Design review of the part built by this model. Coordinates are the model's own, in mm. A direction names the side the tool comes from. Round coordinates to 2 decimals unless told otherwise and drop trailing zeros. Order: outer loops, then holes, each group sorted by start corner. A loop starts at its lowest first (then second) coordinate and runs counter-clockwise, first axis right, second up.
from build123d import *

# Parameters (mm, degrees)
BOSS_EXTRUDE1_DEPTH = 177.8
CUT_EXTRUDE1_REACH  = 236.418
SKETCH3_W           = 0.7874
SKETCH3_H           = 5.8674
FILLET1_R           = 0.15875


with BuildPart() as part:
    # Sketch1 → Boss-Extrude1 (new body)
    with BuildSketch(Plane.XY):
        with BuildLine():
            Line((151.898604, 0.02286), (152.4, 0))
            add(Edge.make_bspline(
                [(152.4, 0), (152.232833718, 0.018502415), (151.571843934, 0.091662545), (150.113999557, 0.2838596), (147.749385864, 0.638650629), (144.555943786, 1.170157002), (140.615360499, 1.859099247), (136.007834995, 2.67146013), (130.806388019, 3.562840017), (125.073826155, 4.486154777), (118.864690135, 5.397753278), (112.233312125, 6.272974236), (105.243489487, 7.106058892), (97.969665406, 7.889319693), (90.492724993, 8.606734858), (82.895253241, 9.240670251), (75.258667902, 9.77749908), (67.662928423, 10.198815718), (60.186827499, 10.49170102), (52.905945954, 10.645080099), (45.891743713, 10.644551806), (39.210681048, 10.486247597), (32.923263797, 10.164412711), (27.083700854, 9.670939726), (21.73719754, 9.016508091), (16.924344759, 8.204081974), (12.676275305, 7.249770479), (9.019815693, 6.174457771), (5.965694819, 5.002018522), (3.544032537, 3.769871526), (1.704834708, 2.531499726), (0.575239506, 1.344737529), (-0.170728015, 0.20310696), (0.337603285, -1.001772228), (1.792943226, -1.546726795), (3.794232235, -2.17716446), (6.643400201, -2.643922316), (10.216110654, -3.041953632), (14.530084187, -3.319872228), (19.533969629, -3.497677255), (25.18692206, -3.577638345), (31.428627275, -3.573848082), (38.191948203, -3.496581442), (45.401595317, -3.349308986), (52.97841726, -3.141841288), (60.83867414, -2.885262261), (68.894988424, -2.587930905), (77.057432025, -2.258882887), (85.235009672, -1.907730283), (93.335426834, -1.550168819), (101.266049649, -1.195465221), (108.93417081, -0.862411006), (116.2464986, -0.557504045), (123.110150899, -0.306936183), (129.431690533, -0.107922528), (135.123521438, 0.027974451), (140.103603919, 0.108900525), (144.29941542, 0.13993859), (147.644768246, 0.124243061), (150.083437285, 0.086502888), (151.399782071, 0.04034956), (151.898604, 0.02286)],
                knots=[0, 0, 0, 0, 0.001635356, 0.006466337, 0.014296592, 0.024884209, 0.037943993, 0.053194137, 0.070376569, 0.089257218, 0.109651763, 0.131396199, 0.15429467, 0.178096903, 0.202530723, 0.227328973, 0.252225807, 0.276966075, 0.301296827, 0.324972089, 0.347773046, 0.369493849, 0.389946985, 0.408979416, 0.42646579, 0.442306729, 0.45642124, 0.468773538, 0.47934515, 0.488155641, 0.495223141, 0.500608248, 0.504417036, 0.507344225, 0.511892731, 0.518766333, 0.5280624, 0.539750485, 0.553781924, 0.570059197, 0.588441486, 0.608747967, 0.630750044, 0.65420771, 0.678865071, 0.70445057, 0.730677503, 0.757253937, 0.783882587, 0.810265561, 0.836095192, 0.861073222, 0.884896986, 0.907258357, 0.92785625, 0.946394646, 0.962618154, 0.976286171, 0.987192828, 0.99514679, 1, 1, 1, 1], degree=3))
        make_face()
    extrude(amount=BOSS_EXTRUDE1_DEPTH)

    # Sketch3 → Cut-Extrude1 (cut, up to next)
    with BuildSketch(Plane.XY.offset(177.8), mode=Mode.PRIVATE) as cut_extrude1_sk1:
        with BuildLine():
            Line((76.2, -2.290863726), (76.2, 9.698555773))
            add(Edge.make_bspline(
                [(76.2, 9.698555773), (75.880486903, 9.71922899), (73.021718792, 9.901577043), (67.662928423, 10.198815718), (60.186827499, 10.49170102), (52.905945954, 10.645080099), (45.891743713, 10.644551806), (39.210681048, 10.486247597), (32.923263797, 10.164412711), (27.083700854, 9.670939726), (21.73719754, 9.016508091), (16.924344759, 8.204081974), (12.676275305, 7.249770479), (9.019815693, 6.174457771), (5.965694819, 5.002018522), (3.544032537, 3.769871526), (1.704834708, 2.531499726), (0.575239506, 1.344737529), (-0.170728015, 0.20310696), (0.337603285, -1.001772228), (1.792943226, -1.546726795), (3.794232235, -2.17716446), (6.643400201, -2.643922316), (10.216110654, -3.041953632), (14.530084187, -3.319872228), (19.533969629, -3.497677255), (25.18692206, -3.577638345), (31.428627275, -3.573848082), (38.191948203, -3.496581442), (45.401595317, -3.349308986), (52.97841726, -3.141841288), (60.83867414, -2.885262261), (68.610964891, -2.598413254), (73.753094803, -2.392038155), (76.2, -2.290863726)],
                knots=[0.249112544, 0.249112544, 0.249112544, 0.249112544, 0.252225807, 0.276966075, 0.301296827, 0.324972089, 0.347773046, 0.369493849, 0.389946985, 0.408979416, 0.42646579, 0.442306729, 0.45642124, 0.468773538, 0.47934515, 0.488155641, 0.495223141, 0.500608248, 0.504417036, 0.507344225, 0.511892731, 0.518766333, 0.5280624, 0.539750485, 0.553781924, 0.570059197, 0.588441486, 0.608747967, 0.630750044, 0.65420771, 0.678865071, 0.70445057, 0.730677503, 0.754490355, 0.754490355, 0.754490355, 0.754490355], degree=3))
        make_face()
    cut_extrude1_tool1 = extrude(cut_extrude1_sk1.sketch, amount=-CUT_EXTRUDE1_REACH, mode=Mode.PRIVATE) & part.part
    # Sketch3 → Cut-Extrude1 (cut, up to next)
    with BuildSketch(Plane.XY.offset(177.8), mode=Mode.PRIVATE) as cut_extrude1_sk2:
        with BuildLine():
            add(Edge.make_bspline(
                [(152.329043318, 0.007856204), (152.185531128, 0.023755853), (151.548249147, 0.094773199), (150.113999557, 0.2838596), (147.749385864, 0.638650629), (144.555943786, 1.170157002), (140.615360499, 1.859099247), (136.007834995, 2.67146013), (130.806388019, 3.562840017), (125.073826155, 4.486154777), (118.864690135, 5.397753278), (112.233312125, 6.272974236), (105.243489487, 7.106058892), (97.969665406, 7.889319693), (90.492724993, 8.606734858), (83.890828887, 9.157599111), (79.789825298, 9.456414677), (78.232, 9.563171971)],
                knots=[0.000231386, 0.000231386, 0.000231386, 0.000231386, 0.001635356, 0.006466337, 0.014296592, 0.024884209, 0.037943993, 0.053194137, 0.070376569, 0.089257218, 0.109651763, 0.131396199, 0.15429467, 0.178096903, 0.202530723, 0.227328973, 0.242511926, 0.242511926, 0.242511926, 0.242511926], degree=3))
            Line((78.232, 9.563171971), (78.232, 6.637546024))
            Line((78.232, 6.637546024), (78.232, 0.770146024))
            Line((78.232, 0.770146024), (78.232, -2.206181248))
            add(Edge.make_bspline(
                [(78.232, -2.206181248), (80.57481261, -2.107809283), (85.628331607, -1.890368614), (93.335426834, -1.550168819), (101.266049649, -1.195465221), (108.93417081, -0.862411006), (116.2464986, -0.557504045), (123.110150899, -0.306936183), (129.431690533, -0.107922528), (135.123521438, 0.027974451), (140.103603919, 0.108900525), (144.29941542, 0.13993859), (147.644768246, 0.124243061), (150.083437285, 0.086502888), (151.399782071, 0.04034956), (151.898604, 0.02286)],
                knots=[0.761082134, 0.761082134, 0.761082134, 0.761082134, 0.783882587, 0.810265561, 0.836095192, 0.861073222, 0.884896986, 0.907258357, 0.92785625, 0.946394646, 0.962618154, 0.976286171, 0.987192828, 0.99514679, 1, 1, 1, 1], degree=3))
            Line((151.898604, 0.02286), (152.4, 0))
            add(Edge.make_bspline(
                [(152.4, 0), (152.376347675, 0.002617903), (152.352695351, 0.005235806), (152.329043318, 0.007856204)],
                knots=[0, 0, 0, 0, 0.000231386, 0.000231386, 0.000231386, 0.000231386], degree=3))
        make_face()
    cut_extrude1_tool2 = extrude(cut_extrude1_sk2.sketch, amount=-CUT_EXTRUDE1_REACH, mode=Mode.PRIVATE) & part.part
    # Sketch3 → Cut-Extrude1 (cut, up to next)
    with BuildSketch(Plane.XY.offset(177.8), mode=Mode.PRIVATE) as cut_extrude1_sk3:
        with Locations((77.8383, 3.703846024)):
            Rectangle(SKETCH3_W, SKETCH3_H)
    cut_extrude1_tool3 = extrude(cut_extrude1_sk3.sketch, amount=-CUT_EXTRUDE1_REACH, mode=Mode.PRIVATE) & part.part
    add(cut_extrude1_tool1.solids().sort_by_distance((41.071648, 3.198464, 177.8))[0], mode=Mode.SUBTRACT)
    add(cut_extrude1_tool2.solids().sort_by_distance((102.964201, 2.96286, 177.8))[0], mode=Mode.SUBTRACT)
    add(cut_extrude1_tool3.solids().sort_by_distance((77.8383, 3.703846, 177.8))[0], mode=Mode.SUBTRACT)

    # Fillet1
    fillet1_edges = [part.edges().sort_by_distance(p)[0] for p in [
        (78.232, -2.206181248, 88.9),
        (78.232, 9.563171971, 88.9),
        (78.232, 0.770146024, 88.9),
        (77.4446, 0.770146024, 88.9),
        (78.232, 6.637546024, 88.9),
        (77.4446, 6.637546024, 88.9),
    ]]
    fillet(fillet1_edges, radius=FILLET1_R)


solid = part.part
1) Clearance check with flat-ended pins moving along their axes: P1, Ø3, axis at y = 3, z = 88.5, coming from the +X side; P2, Ø1, axis at x = 76.5, y = 0, coming from the -Z side; P3, Ø0.5, axis at x = 78, z = 117, coming from the -Y side. State where each tip first meets the part, or that it passes through.
Results:
P1: stops at x = 77.44
P2: stops at z = 0
P3: stops at y = -2.23
2) Take a section at A-A on y = 4.25. Give the boundary of the cut face in (x, z).
Results:
outline: (76.2, 0) - (77.44, 0) - (77.44, 177.8) - (76.2, 177.8) - close
3) For faces 1 (the face through (77.445, 4, 90)), 2 (the face through (76.2, 4, 90)), list the 3-axis set-ups (+Z, -Z, +X, -X, +Y, -Y) from which the entire face can be reached by the end or side of a thin tool; tool diameter is ignored.
Results:
face 1: +Z, -Z, +X
face 2: +Z, -Z, -X, +Y, -Y
4) To check wall thickness, follow line 1 along Y through (x, z) = (77.95, 76); line 2 along X through (y, z) = (1, 139); line 3 along Y through (x, z) = (76.55, 36). State the ranges of each line that lie inside material, in increasing order.
Results:
line 1: y = -2.22 to 0.77, 6.64 to 9.58
line 2: x = 76.2 to 77.44
line 3: y = -2.28 to 9.68
